Design review of the part built by this model. Coordinates are the model's own, in mm. Face numbers are marked on the shaded views. Round coordinates to 2 decimals unless told otherwise and drop trailing zeros. Order: outer loops, then holes, each group sorted by start corner. A loop starts at its lowest first (then second) coordinate and runs counter-clockwise, first axis right, second up. Notation, with made-up numbers: (75.25, 89.25) - (125.25, 89.25) arc R18 cw to (125.25, 103.25) - close; hole circle Ø7 at (63, 60.25). An arc over 180 degrees is marked (long way). Write item = value, one per line.
Autodesk Inventor part; units mm, degrees
ref_plane "YZ Plane" through (0, 0, 0) normal (1, 0, 0) x (0, 1, 0)
ref_plane "XZ Plane" through (0, 0, 0) normal (0, 1, 0) x (-1, 0, 0)
ref_plane "XY Plane" through (0, 0, 0) normal (0, 0, 1) x (1, 0, 0)
sketch "Skizze1" plane through (0, 0, 0) normal (0, 0, 1) x (1, 0, 0)
  line L0 (0, 0) -> (230, 0)
  line L1 (230, 0) -> (230, 180)
  line L2 (230, 180) -> (0, 180)
  line L3 (0, 180) -> (0, 0)
  dimension "d0" = 230
  dimension "d1" = 180
extrude "Grobblech1" add sketch "Skizze1" along normal blind 2
sketch "Skizze2" plane through (230, 2, 0) normal (0, -1, 0) x (1, 0, 0)
  line L0 (-230, 0) -> (0, 0)
  line L1 (0, 0) -> (0, 20)
  line L2 (0, 20) -> (-230, 20)
  line L3 (-230, 20) -> (-230, 0)
edge flange "Lasche1" height 20 angle 90 thickness 2 bend radius 2 thickness toward (0, -1, 0) relief tear relief width 2 relief depth 1 corner gap 2 corner form 0 edges at (115, 0, 2) (115, 180, 2) wall of the first edge with corners at (0, 2, 0) (230, 2, 0) (230, 2, 20) (0, 2, 20)
bend "Biegung1"
corner "Ecke1"
sketch "Skizze3" plane through (0, 0, 0) normal (0, 0, -1) x (-1, 0, 0)
  circle A0 centre (-36.5, 97.5) radius 1.621
  circle A1 centre (-36.5, 82.5) radius 1.621
  circle A2 centre (-193.5, 97.5) radius 1.621
  circle A3 centre (-193.5, 82.5) radius 1.621
  line L0 (0, 0) -> (-36.5, 0)
  line L1 (-36.5, 0) -> (-36.5, 82.5)
  line L2 (-36.5, 82.5) -> (0, 82.5)
  line L3 (0, 82.5) -> (0, 0)
  line L4 (-36.5, 82.5) -> (-193.5, 82.5)
  line L5 (-193.5, 82.5) -> (-193.5, 97.5)
  line L6 (-193.5, 97.5) -> (-36.5, 97.5)
  line L7 (-36.5, 97.5) -> (-36.5, 82.5)
  circle A4 centre (-115, 97.5) radius 1.621
  circle A5 centre (-115, 82.5) radius 1.621
hole "Bohrung1" at (115, 97.5, 0) at (115, 82.5, 0) direction (0, 0, 1) diameter 4 depth 2 tip angle 118
fillet "Eckenrundung1" radius 3 4 edges at (230, 1, 20) (230, 179, 20) (0, 179, 20) (0, 1, 20)
equation "\"d19\" = Stärke"
equation "\"d2\" = Stärke"
equation "\"d3\" = BreiteBiegungsfreistellung"
equation "\"d4\" = TiefeBiegungsfreistellung"
equation "\"d5\" = MinimalRest"
equation "\"d6\" = Übergangsradius"
equation "\"d9\" = Biegeradius"
equation "\"d10\" = GrößeEckenfreistellung"
equation "\"d11\" = Abstandsgröße"
equation "\"d12\" = JacobiRadiusGröße"
equation "\"Biegeradius\" = Stärke"
equation "\"BreiteBiegungsfreistellung\" = Stärke"
equation "\"TiefeBiegungsfreistellung\" = 0.5 * Stärke"
equation "\"GrößeEckenfreistellung\" = 4 * Stärke"
equation "\"MinimalRest\" = 2 * Stärke"
equation "\"Übergangsradius\" = Biegeradius"
equation "\"JacobiRadiusGröße\" = Biegeradius"
equation "\"Abstandsgröße\" = Stärke"
properties part number "Schale"
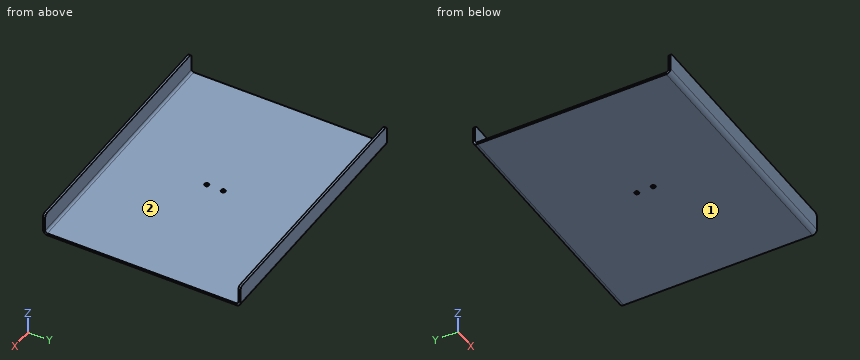
1) Clearance check with flat-ended pins moving along their axes: pin 1 Ø4 at (x, y) = (26, 102.5) entering from +Z; pin 2 Ø3.5 at (x, y) = (115, 97.5) entering from +Z. State where each tip first meets the part, or that it passes through.
Findings:
pin_1 = 2
pin_2 = through
2) We need section B-B on x = 15. Write out the cut boundary in (y, z), and give its area (3 significant figures).
Findings:
outline = (0, 4) arc R4 ccw to (4, 0) - (176, 0) arc R4 ccw to (180, 4) - (180, 20) - (178, 20) - (178, 4) arc R2 cw to (176, 2) - (4, 2) arc R2 cw to (2, 4) - (2, 20) - (0, 20) - close
area = 427 mm^2
3) To check wall thickness, follow L1, parallel to Y at x = 207.5, z = 13; L2, parallel to Y at x = 115, z = 1.4; L3, parallel to Y at x = 115, z = 0.8. State the ranges of each line that lie inside material, in increasing order. Write a range as from..to.
Findings:
L1 = 0..2, 178..180
L2 = 0.96..80.5, 84.5..95.5, 99.5..179.04
L3 = 1.6..80.5, 84.5..95.5, 99.5..178.4
4) The part is to be moulded in two halves that separate along Y. For the marked faces 1 and 2, say which applies: released by +Y, released by -Y, zero draft, split by the parting line, or undercut.
Findings:
face_1 = zero draft
face_2 = undercut
5) We need section A-A on z = 8. Write out the cut boundary in (x, y).
Findings:
outline = (0, 0) - (230, 0) - (230, 2) - (0, 2) - close; (0, 178) - (230, 178) - (230, 180) - (0, 180) - close
6) We need section C-C on y = 77. Write out the cut boundary in (x, z), and give its area (3 significant figures).
Findings:
outline = (0, 0) - (230, 0) - (230, 2) - (0, 2) - close
area = 460 mm^2
